Part model, mm, in its own coordinate system. Give positions to 0.01 mm unless a question says otherwise; leave off trailing zeros. Order: outer loops, then holes, each group sorted by start corner. A loop starts at its lowest first (then second) coordinate and runs counter-clockwise, first axis right, second up. Notation, with made-up numbers: (-7.5, 53.25) -> (33.5, 53.25) arc R32 ccw to (33.5, 86.25) -> close; hole circle Ø8 at (71, 29). An arc over 180 degrees is marked (long way). Write item = value, one per line. Start each with the question number.
(1) Probe line 1 along X through (y, z) = (2.3, 0); line 2 along Z through (x, y) = (0, 0.8); line 3 along X through (y, z) = (2.55, 0.5). List the from-to ranges inside material, lowest first. Write a range as from..to.
(2) Saw through at A-A, the plane x = 0. List the corners of the cut face in (y, z).
(3) Saw through at D-D, the plane z = 7. List the corners of the cut face in (x, y), then the cut area to 3 significant figures.
(4) Saw through at B-B, the plane z = -2. List the corners of the cut face in (x, y), then the cut area to 3 significant figures.
(5) Saw through at C-C, the plane y = 0.6. List the corners of the cut face in (x, z), then the cut area to 3 significant figures.
(6) Two-plate mould, pull along Z, no slides. Class faces 1 (the cylindrical face through (-4.64, 1.97, 8.95)), 2 (the cylindrical face through (14.985, 1.972, -0.66)), 3 (the flat face through (0.2, 4, -6.5)): pulls with the +Z half, pulls with the -Z half, needs draft (parallel to the pull), parting line crosses it, or undercut.
(7) Flat gauge pin, fed straight in: pin 1 (1.5 mm diameter, centred on x = -10.5, y = 2.5, fed in from -Z). Where does the tip first touch, or does it go through?
Autodesk Inventor part; units mm, degrees
ref_plane "YZ Plane" through (0, 0, 0) normal (1, 0, 0) x (0, 1, 0)
ref_plane "XZ Plane" through (0, 0, 0) normal (0, 1, 0) x (-1, 0, 0)
ref_plane "XY Plane" through (0, 0, 0) normal (0, 0, 1) x (1, 0, 0)
sketch "Skizze1" plane through (0, 0, 0) normal (0, 1, 0) x (-1, 0, 0)
  circle A0 centre (0, 0) radius 15
  circle A1 centre (0, 0) radius 6
  circle A2 centre (0, 0) radius 11.5
  line L0 (0, 0) -> (-26.7883, 0)
  line L1 (0, 0) -> (13.3942, -23.1994)
  line L2 (0, 0) -> (13.3942, 23.1994)
  circle A3 centre (5.75, -9.9593) radius 1.5
  circle A4 centre (5.75, 9.9593) radius 1.5
  circle A5 centre (-11.5, 0) radius 1.5
  dimension "d0" = 30
  dimension "d1" = 12
  dimension "d3" = 23
  dimension "d6" = 360
  dimension "d8" = 3
  dimension "d9" = 3
  dimension "d10" = 3
extrude "Extrusion1" add sketch "Skizze1" along normal blind 4 contours A0 L1 A3 A2 A4 L2 | L2 A4 A2 A5 L0 A0 | A0 L0 A5 A2 A3 L1 | A4 L2 A1 L0 A5 A2 | A2 A5 L0 A1 L1 A3 | A2 A3 L1 A1 L2 A4
properties part number "01-03-01-02 Zeichnung Zange links oben"
Results list:
q1.line_1 = -15..-6, 6..10, 13..15
q1.line_2 = -15..-6, 6..15
q1.line_3 = -14.99..-5.98, 5.98..10.09, 12.91..14.99
q2.outline = (0, -15) -> (4, -15) -> (4, -6) -> (0, -6) -> close; (0, 6) -> (4, 6) -> (4, 15) -> (0, 15) -> close
q3.outline = (-13.27, 0) -> (13.27, 0) -> (13.27, 4) -> (-13.27, 4) -> close
q3.area = 106 mm^2
q4.outline = (-14.87, 0) -> (-5.66, 0) -> (-5.66, 4) -> (-14.87, 4) -> close; (5.66, 0) -> (14.87, 0) -> (14.87, 4) -> (5.66, 4) -> close
q4.area = 73.7 mm^2
q5.outline = circle Ø30 at (0, 0); hole circle Ø3 at (-5.75, -9.96); hole circle Ø3 at (-5.75, 9.96); hole circle Ø12 at (0, 0); hole circle Ø3 at (11.5, 0)
q5.area = 573 mm^2
q6.face_1 = undercut
q6.face_2 = parting line crosses it
q6.face_3 = needs draft
q7.pin_1 = -11.4
